Source: CAD feature listing. Evaluate the final solid. Frame: model axes, mm. Coordinates: 2 decimals unless noted, no trailing zeros. Loops run counter-clockwise (first coordinate to the right, second up) from the corner with the lowest first, then second, coordinate; pieces in that order, holes last.
from build123d import *

# Parameters (mm, degrees)
SKETCH2_R               = 3.175
BOSS_EXTRUDE1_DEPTH     = 50
SKETCH3_R               = 3.175
BOSS_EXTRUDE2_DEPTH     = 3.175
SKETCH5_R               = 0.5953125
CUT_EXTRUDE1_DEPTH      = 4.175
CUT_EXTRUDE1_DEPTH_BACK = 4.175


with BuildPart() as part:
    # Sketch2 → Boss-Extrude1 (new body)
    with BuildSketch(Plane.XY):
        Circle(SKETCH2_R)
    boss_extrude1 = extrude(amount=BOSS_EXTRUDE1_DEPTH)

    # Sketch3 → Boss-Extrude2 (add)
    with BuildSketch(Plane.XY.offset(50)):
        Circle(SKETCH3_R)
    boss_extrude2 = extrude(amount=BOSS_EXTRUDE2_DEPTH)

    # Mirror1: Boss-Extrude1, Boss-Extrude2 across plane
    add(boss_extrude1.mirror(Plane.XY))
    add(boss_extrude2.mirror(Plane.XY))

    # Sketch5 → Cut-Extrude1 (cut, two sides)
    with BuildSketch(Plane(origin=(0, 0, 0), x_dir=(0, 0, -1), z_dir=(1, 0, 0))) as cut_extrude1_sk:
        with Locations((-51.5875, 0)):
            Circle(SKETCH5_R)
        with Locations((51.5875, 0)):
            Circle(SKETCH5_R)
    extrude(amount=CUT_EXTRUDE1_DEPTH, mode=Mode.SUBTRACT)
    extrude(cut_extrude1_sk.sketch, amount=-CUT_EXTRUDE1_DEPTH_BACK, mode=Mode.SUBTRACT)


solid = part.part
Q1. Section C-C, the plane y = -1.75. Return the cut outline in (x, z) (3 decimals).
Q2. Contact query for a flat-ended pin moving along its axis: pin 1 Ø1 at (y, z) = (0, -51.59) entering from +X. Output: stop coordinate, or through.
Q3. Line query: line 1 along Z through (x, y) = (1.2, 0) (3 decimals); line 2 along Z through (x, y) = (-0.25, -0.5) (3 decimals); line 3 along Y through (x, z) = (-0.25, -21). Output: solid intervals per line, ascending.
Q4. Section B-B, the plane x = 1.5. Return the cut outline in (y, z) (1 decimal), plus the area to 3 significant figures.
Q5. Section A-A, the plane z = -16.5. Return the cut outline in (x, y) (3 decimals), plus the area to 3 significant figures.
Derived:
1. outline: (-2.649, -53.175) - (2.649, -53.175) - (2.649, 53.175) - (-2.649, 53.175) - close
2. pin 1: passes through
3. line 1: z = -53.175 to -52.183, -50.992 to 50.992, 52.183 to 53.175
3. line 2: z = -53.175 to -51.911, -51.264 to 51.264, 51.911 to 53.175
3. line 3: y = -3.17 to 3.17
4. outline: (-2.8, -53.2) - (2.8, -53.2) - (2.8, 53.2) - (-2.8, 53.2) - close; hole circle Ø1.2 at (0, -51.6); hole circle Ø1.2 at (0, 51.6)
4. area: 593 mm2
5. outline: circle Ø6.35 at (0, 0)
5. area: 31.7 mm2
